Autodesk Inventor part; units mm, degrees
ref_plane "YZ Plane" through (0, 0, 0) normal (1, 0, 0) x (0, 1, 0)
ref_plane "XZ Plane" through (0, 0, 0) normal (0, 1, 0) x (-1, 0, 0)
ref_plane "XY Plane" through (0, 0, 0) normal (0, 0, 1) x (1, 0, 0)
sketch "Sketch1" plane through (0, 0, 0) normal (0, 0, 1) x (1, 0, 0)
  line L0 (0, 0) -> (25.4, 0)
  line L1 (25.4, 0) -> (25.4, 25.4)
  line L2 (25.4, 25.4) -> (0, 25.4)
  line L3 (0, 25.4) -> (0, 0)
  line L4 (3.175, 3.175) -> (22.225, 3.175)
  line L5 (22.225, 3.175) -> (22.225, 22.225)
  line L6 (22.225, 22.225) -> (3.175, 22.225)
  line L7 (3.175, 22.225) -> (3.175, 3.175)
  dimension "d0" = 25.4
  dimension "d1" = 25.4
  dimension "d2" = 19.05
  dimension "d3" = 19.05
  dimension "d4" = 3.175
  dimension "d5" = 3.175
extrude "Extrusion1" add sketch "Sketch1" along normal blind 304.8
sketch "Sketch2" plane through (0, 25.4, 0) normal (0, 1, 0) x (1, 0, 0)
  line L0 (25.4, 0) -> (0, 0)
  line L1 (0, 0) -> (0, -304.8)
  line L2 (25.4, -304.8) -> (0, -304.8)
  line L3 (25.4, 0) -> (25.4, -304.8)
  point P0 (12.7, -292.1)
  point P1 (12.7, -12.7)
  point P2 (12.7, -165.1)
  dimension "d8" = 12.7
  dimension "d9" = 12.7
  dimension "d10" = 12.7
  dimension "d11" = 12.7
  dimension "d32" = 12.7
  dimension "d33" = 139.7
sketch "Sketch3" plane through (25.4, 0, 0) normal (1, 0, 0) x (0, 0, -1)
  line L0 (0, 0) -> (-304.8, 0)
  line L1 (0, 0) -> (0, 25.4)
  point P0 (-38.1, 12.7)
  point P1 (-63.5, 12.7)
  point P2 (-88.9, 12.7)
  dimension "d19" = 12.7
  dimension "d20" = 12.7
  dimension "d21" = 12.7
  dimension "d22" = 38.1
  dimension "d23" = 88.9
  dimension "d24" = 63.5
hole "Hole2" at (25.4, 12.7, 38.1) at (25.4, 12.7, 63.5) at (25.4, 12.7, 88.9) direction (-1, 0, 0) diameter 6.35 end through all
hole "Hole3" at (12.7, 25.4, 292.1) at (12.7, 25.4, 12.7) at (12.7, 25.4, 165.1) direction (0, -1, 0) diameter 6.35 end through all
sketch "Sketch4" plane through (25.4, 0, 0) normal (1, 0, 0) x (0, 0, -1)
  circle A0 centre (-63.5, 12.7) radius 3.175
  circle A1 centre (-38.1, 12.7) radius 3.175
  circle A2 centre (-88.9, 12.7) radius 3.175
  line L0 (0, 0) -> (0, 25.4)
  line L1 (0, 25.4) -> (-304.8, 25.4)
  line L2 (-304.8, 0) -> (-304.8, 25.4)
  line L3 (0, 0) -> (-304.8, 0)
  point P0 (-177.8, 12.7)
  point P1 (-114.3, 12.7)
  point P2 (-152.4, 12.7)
  dimension "d41" = 127
  dimension "d42" = 190.5
  dimension "d43" = 152.4
  dimension "d44" = 12.7
  dimension "d45" = 12.7
  dimension "d46" = 12.7
hole "Hole4" at (25.4, 12.7, 177.8) at (25.4, 12.7, 114.3) at (25.4, 12.7, 152.4) direction (-1, 0, 0) diameter 6.35 end through all
sketch "Sketch5" plane through (0, 0, 304.8) normal (0, 0, 1) x (1, 0, 0)
  line L0 (3.175, 3.175) -> (3.175, 22.225)
  line L1 (3.175, 22.225) -> (22.225, 22.225)
  line L2 (22.225, 22.225) -> (22.225, 3.175)
  line L3 (22.225, 3.175) -> (3.175, 3.175)
  line L4 (0, 0) -> (25.4, 0)
  line L5 (25.4, 0) -> (25.4, 25.4)
  line L6 (25.4, 25.4) -> (0, 25.4)
  line L7 (0, 25.4) -> (0, 0)
extrude "Extrusion2" add sketch "Sketch5" along normal blind 177.8
sketch "Sketch6" plane through (0, 25.4, 0) normal (0, 1, 0) x (1, 0, 0)
  line L0 (25.4, -482.6) -> (0, -482.6)
  line L1 (25.4, 0) -> (25.4, -482.6)
  point P0 (12.7, -469.9)
  point P1 (12.7, -419.1)
  dimension "d56" = 12.7
  dimension "d57" = 12.7
  dimension "d65" = 63.5
  dimension "d66" = 12.7
hole "Hole6" at (12.7, 25.4, 469.9) at (12.7, 25.4, 419.1) direction (0, -1, 0) diameter 6.35 depth 25.4 tip angle 118
sketch "Sketch7" plane through (0, 25.4, 0) normal (0, 1, 0) x (1, 0, 0)
  circle A0 centre (12.7, -469.9) radius 3.175
  circle A1 centre (12.7, -419.1) radius 3.175
  circle A2 centre (12.7, -12.7) radius 3.175
  circle A3 centre (12.7, -292.1) radius 3.175
  circle A4 centre (12.7, -165.1) radius 3.175
  line L0 (25.4, 0) -> (0, 0)
  line L1 (0, 0) -> (0, -482.6)
  line L2 (25.4, -482.6) -> (0, -482.6)
  line L3 (25.4, 0) -> (25.4, -482.6)
  point P0 (12.7, -393.7)
  point P1 (12.7, -317.5)
  dimension "d74" = 12.7
  dimension "d75" = 12.7
  dimension "d76" = 88.9
  dimension "d77" = 165.1
hole "Hole7" at (12.7, 25.4, 393.7) at (12.7, 25.4, 317.5) direction (0, -1, 0) diameter 6.35 end through all
properties part number "mounting block" material "Aluminum 6061"
For this review, take the finished solid that the model builds, in its own axes (mm). A direction names the side the tool comes from. Coordinates: 2 decimals unless noted, no trailing zeros. Order: outer loops, then holes, each group sorted by start corner. A loop starts at its lowest first (then second) coordinate and runs counter-clockwise, first axis right, second up. Notation, with made-up numbers: (44.25, 30) - (65.25, 30) arc R26 ccw to (65.25, 56) - close; hole circle Ø6 at (-21, -13.5). An arc over 180 degrees is marked (long way). Answer as a JSON object with one key per item and string values. Group by question number.
1. We need section A-A on z = 198.5. State the section outline as (x, y) points (3 decimals), then the cut area to 3 significant figures.
2. For faces 4 (the flat face through (0, 13, 238)), 5 (the flat face through (3.175, 13, 238)), list the 3-axis set-ups (+Z, -Z, +X, -X, +Y, -Y) from which the entire face can be reached by the end or side of a thin tool; tool diameter is ignored.
3. For probe 1 along Y at (x, z) = (8, 153.5) (3 decimals); probe 2 along X at (y, z) = (23.7, 419.1) (3 decimals), list the stretches that pass through material, from the lowest coordinate up.
4. The part is to be moulded in two halves that separate along X. For faces 1 (the flat face through (13, 3.175, 238)), 2 (the flat face through (13, 0, 238)), 3 (the flat face through (25.4, 13, 238)), say which applies: pulls with the +X half, pulls with the -X half, needs draft (parallel to the pull), parting line crosses it, or undercut.
5. Clearance check with a flat-ended pin moving along its axis: P1, Ø1.5, axis at y = 18, z = 273.5, coming from the -X side. State where the tip first meets the part, or that it passes through.
Final values:
{
 "1": {"outline": "(0, 0) - (25.4, 0) - (25.4, 25.4) - (0, 25.4) - close; hole (3.175, 3.175) - (22.225, 3.175) - (22.225, 22.225) - (3.175, 22.225) - close", "area": "282 mm²"},
 "2": {"face 4": "+Z, -Z, -X, +Y, -Y", "face 5": "+Z, -Z"},
 "3": {"probe 1": "0 to 3.175, 22.225 to 25.4", "probe 2": "0 to 9.525, 15.875 to 25.4"},
 "4": {"face 1": "undercut", "face 2": "needs draft", "face 3": "pulls with the +X half"},
 "5": {"P1": "x = 0"}
}
